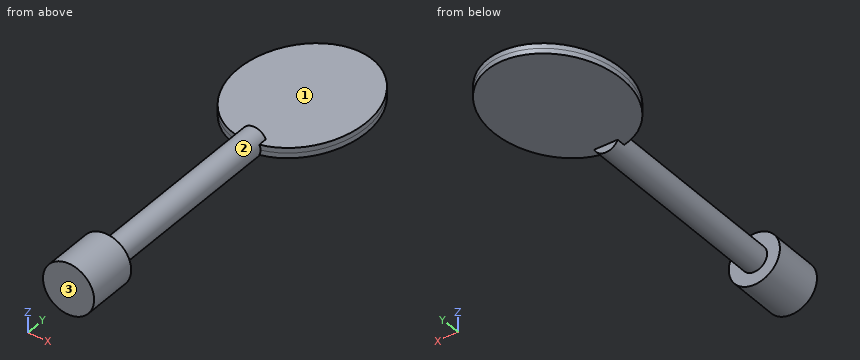
from build123d import *

# Parameters (mm, degrees)
SKETCH_1_R      = 50
EXTRUDE_1_DEPTH = 100
SKETCH_2_R      = 25
EXTRUDE_2_DEPTH = 400
SKETCH_3_RX     = 150
SKETCH_3_RY     = 125
EXTRUDE_3_DEPTH = 10


with BuildPart() as part:
    # 草图1 → 凸台-拉伸1 (new body)
    with BuildSketch(Plane(origin=(0, 0, 0), x_dir=(1, 0, 0), z_dir=(0, 1, 0))):
        with Locations(Location((0, 0, 0), (0, 0, 270))):
            Circle(SKETCH_1_R)
    extrude(amount=EXTRUDE_1_DEPTH)

    # 草图2 → 凸台-拉伸2 (add)
    with BuildSketch(Plane(origin=(0, 100, 0), x_dir=(1, 0, 0), z_dir=(0, 1, 0))):
        with Locations(Location((0, 0, 0), (0, 0, 270))):
            Circle(SKETCH_2_R)
    extrude(amount=EXTRUDE_2_DEPTH)

    # 草图3 → 凸台-拉伸3 (add, symmetric)
    with BuildSketch(Plane.XY):
        with Locations(Location((0, 630), (0, 0, 90))):
            Ellipse(SKETCH_3_RX, SKETCH_3_RY)
    extrude(amount=EXTRUDE_3_DEPTH, both=True)


solid = part.part
The model under review builds one solid part; all positions refer to its coordinate system, in mm. Face numbers are marked on the shaded views. Round coordinates to 2 decimals unless told otherwise and drop trailing zeros. Loops run counter-clockwise (first coordinate to the right, second up) from the corner with the lowest first, then second, coordinate; pieces in that order, holes last. Notation, with made-up numbers: M 30.5,27.5 L 40.5,27.5 A12 ccw 40.5,50.5 Z; hole C 0,58.5 d10. An arc over 180 degrees is marked long. Answer as CSV lines item,"result".
1. Draft analysis for pull direction Y (two halves, no side actions). For the marked faces 1, 2 and 3, state which applies: pulls with the +Y half, pulls with the -Y half, needs draft (parallel to the pull), parting line crosses it, or undercut.
Outcome:
face 1,"needs draft"
face 2,"undercut"
face 3,"pulls with the -Y half"
2. To check wall thickness, follow L1, parallel to Y at x = 33, z = -22.5; L2, parallel to Z at x = 31, y = 687; L3, parallel to X at y = 32, z = -14.5. State the ranges of each line that lie inside material, in increasing order. Write a range as [from, to].
Outcome:
L1,"y = [0, 100]"
L2,"z = [-10, 10]"
L3,"x = [-47.85, 47.85]"
3. We need section C-C (z = -43). Give the boundary of the cut face in (x, y), plus the area to 3 significant figures.
Outcome:
outline,"M -25.51,0 L 25.51,0 L 25.51,100 L -25.51,100 Z"
area,"5,100 mm2"
4. We need section A-A (z = 18). Give the boundary of the cut face in (x, y), plus the area to 3 significant figures.
Outcome:
outline,"M -46.65,0 L 46.65,0 L 46.65,100 L 17.35,100 L 17.35,500 L -17.35,500 L -17.35,100 L -46.65,100 Z"
area,"23,200 mm2"
5. We need section B-B (y = 118). Give the boundary of the cut face in (x, z), plus the area to 3 significant figures.
Outcome:
outline,"C 0,0 d50"
area,"1,960 mm2"
6. Insertion check: pin 1 Ø8 at (y, z) = (314, -20) entering from +X; pin 2 Ø3 at (x, y) = (-26, 671) entering from -Z; pin 3 Ø5 at (x, y) = (-38.5, 573.5) entering from +Z. Each pin has a flat end and moves straight along its axis. Give the tip position at first contact, or say it passes through.
Outcome:
pin 1,"stops at x = 19.21"
pin 2,"stops at z = -10"
pin 3,"stops at z = 10"
